Geometry check sheet. Reference: the model listing, model coordinates, mm. Face numbers are marked on the shaded views. A direction names the side the tool comes from. Round coordinates to 2 decimals unless told otherwise and drop trailing zeros. Loops run counter-clockwise (first coordinate to the right, second up) from the corner with the lowest first, then second, coordinate; pieces in that order, holes last. Notation, with made-up numbers: (-12, 68.5) - (-7, 68.5) arc R29 ccw to (-7, 100.5) - close; hole circle Ø7 at (75.5, -24.75). An arc over 180 degrees is marked (long way). Write item = value, one per line.
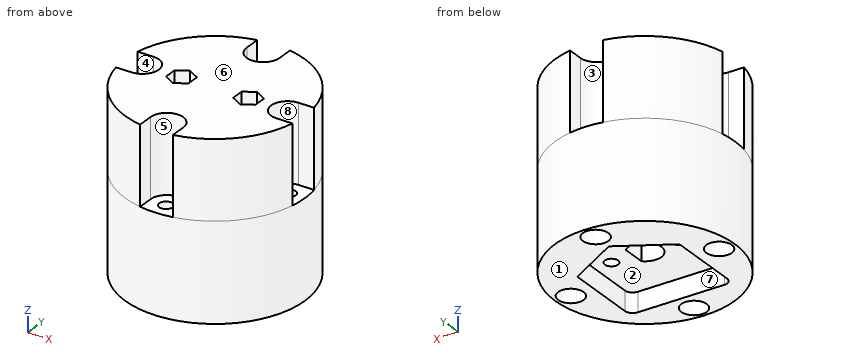
```python
from build123d import *

# Parameters (mm, degrees)
BOSS_EXTRUDE1_OUTLINE_R    = 16
BOSS_EXTRUDE1_DEPTH        = 15
SKETCH2_W                  = 7.4
SKETCH2_H                  = 24.742483552
CUT_EXTRUDE1_DEPTH         = 16.8
SKETCH3_R                  = 1.71
CUT_EXTRUDE2_DEPTH         = 70
BOSS_EXTRUDE2_DEPTH        = 20
BOSS_EXTRUDE2_DEPTH_BACK   = 5
SKETCH10_R                 = 23
SKETCH10_R_2               = 1.7
CUT_EXTRUDE4_DEPTH         = 25
SKETCH3_11_R               = 1.71
CUT_EXTRUDE5_DEPTH         = 55
CUT_EXTRUDE6_DEPTH         = 2.3
CUT_EXTRUDE6_DEPTH_BACK    = 0.7
SKETCH14_R                 = 12.3
BOSS_EXTRUDE3_START        = 20
BOSS_EXTRUDE3_DEPTH        = 20
SKETCH19_R                 = 16.2
CUT_EXTRUDE7_DEPTH         = 2.2
CUT_EXTRUDE8_START         = 35
CUT_EXTRUDE8_OUTLINE_R     = 1.7
CUT_EXTRUDE8_DEPTH         = 20
CUT_EXTRUDE9_START         = 2
CUT_EXTRUDE9_OUTLINE_R     = 16
CUT_EXTRUDE9_OUTLINE_R_2   = 15.484452344
CUT_EXTRUDE9_DEPTH         = 8
CUT_EXTRUDE9_START_2       = 10
CUT_EXTRUDE9_2_OUTLINE_R   = 3.25
CUT_EXTRUDE9_2_OUTLINE_R_2 = 1.7
CUT_EXTRUDE9_2_DEPTH       = 3
CUT_EXTRUDE10_DEPTH        = 3.6
SKETCH36_R                 = 15.484452344
CUT_EXTRUDE11_DEPTH        = 8
CUT_EXTRUDE13_DEPTH        = 5
CUT_EXTRUDE14_DEPTH        = 10
SKETCH39_R                 = 3.25
CUT_EXTRUDE15_DEPTH        = 5


# Read off the part's stored shape, not the designer's step: Boss-Extrude1, Cut-Extrude8, Cut-Extrude9
with BuildPart() as part:
    # Boss-Extrude1 outline → Boss-Extrude1 (new body)
    with BuildSketch(Plane(origin=(0, 0, 0), x_dir=(0, 1, 0), z_dir=(0, 0, 1))):
        Circle(BOSS_EXTRUDE1_OUTLINE_R)
    extrude(amount=BOSS_EXTRUDE1_DEPTH)

    # Sketch2 → Cut-Extrude1 (cut)
    with BuildSketch(Plane.ZY.offset(16)):
        with Locations((10.1, 0)):
            Rectangle(SKETCH2_W, SKETCH2_H)
    extrude(amount=-CUT_EXTRUDE1_DEPTH, mode=Mode.SUBTRACT)

    # Sketch3 → Cut-Extrude2 (cut)
    with BuildSketch(Plane(origin=(0, 0, 0), x_dir=(0, 1, 0), z_dir=(0, 0, 1))):
        with Locations((0, 8.6)):
            Circle(SKETCH3_R)
    extrude(amount=CUT_EXTRUDE2_DEPTH, mode=Mode.SUBTRACT)

    # Sketch10 → Boss-Extrude2 (add, two sides: drawn at the far end of the back side and taken through both)
    with BuildSketch(Plane(origin=(0, 0, 15), x_dir=(0, 1, 0), z_dir=(0, 0, 1)).offset(-BOSS_EXTRUDE2_DEPTH_BACK)):
        with Locations(Location((0, 0, 0), (0, 0, 270))):
            Circle(SKETCH10_R)
        with Locations(Location((0, 8.6, 0), (0, 0, 270))):
            Circle(SKETCH10_R_2, mode=Mode.SUBTRACT)
        with Locations(Location((0, 19, 0), (0, 0, 270))):
            Circle(SKETCH10_R_2, mode=Mode.SUBTRACT)
        with Locations(Location((18.999966339, -0.035764812, 0), (0, 0, 90))):
            Circle(SKETCH10_R_2, mode=Mode.SUBTRACT)
        with Locations(Location((0, -19, 0), (0, 0, 90))):
            Circle(SKETCH10_R_2, mode=Mode.SUBTRACT)
        with Locations(Location((-18.999966339, -0.035764812, 0), (0, 0, 270))):
            Circle(SKETCH10_R_2, mode=Mode.SUBTRACT)
        with Locations(Location((0, -8.6, 0), (0, 0, 270))):
            Circle(SKETCH10_R_2, mode=Mode.SUBTRACT)
    extrude(amount=BOSS_EXTRUDE2_DEPTH + BOSS_EXTRUDE2_DEPTH_BACK)

    # Sketch3<6> → Cut-Extrude4 (cut)
    with BuildSketch(Plane(origin=(0, 0, 0), x_dir=(0, 1, 0), z_dir=(0, 0, 1))):
        with BuildLine():
            Line((3, -2.939387691), (-3, -2.939387691))
            ThreePointArc((-3, -2.939387691), (0, 4.2), (3, -2.939387691))
        make_face()
    extrude(amount=CUT_EXTRUDE4_DEPTH, mode=Mode.SUBTRACT)

    # Sketch3<11> → Cut-Extrude5 (cut)
    with BuildSketch(Plane(origin=(0, 0, 0), x_dir=(0, 1, 0), z_dir=(0, 0, 1))):
        with Locations(Location((0, -8.6, 0), (0, 0, 90))):
            Circle(SKETCH3_11_R)
    extrude(amount=CUT_EXTRUDE5_DEPTH, mode=Mode.SUBTRACT)

    # Sketch14 → Cut-Extrude6 (cut, two sides: drawn at the far end of the back side and taken through both)
    with BuildSketch(Plane(origin=(0, 0, 7.5), x_dir=(0, 1, 0), z_dir=(0, 0, 1)).offset(-CUT_EXTRUDE6_DEPTH_BACK)):
        Circle(SKETCH14_R)
    extrude(amount=CUT_EXTRUDE6_DEPTH + CUT_EXTRUDE6_DEPTH_BACK, mode=Mode.SUBTRACT)

    # Sketch15 → Boss-Extrude3 (add)
    with BuildSketch(Plane(origin=(0, 0, 35), x_dir=(0, 1, 0), z_dir=(0, 0, 1)).offset(BOSS_EXTRUDE3_START)):
        with BuildLine():
            Line((-4.2, 18.6), (-4.2, 22.61327044))
            ThreePointArc((-4.2, 22.61327044), (-16.263455967, 16.263455967), (-22.61327044, 4.2))
            Line((-22.61327044, 4.2), (-18.6, 4.2))
            ThreePointArc((-18.6, 4.2), (-14.4, 0), (-18.6, -4.2))
            Line((-18.6, -4.2), (-22.61327044, -4.2))
            ThreePointArc((-22.61327044, -4.2), (-16.263455967, -16.263455967), (-4.2, -22.61327044))
            Line((-4.2, -22.61327044), (-4.2, -18.6))
            ThreePointArc((-4.2, -18.6), (0, -14.4), (4.2, -18.6))
            Line((4.2, -18.6), (4.2, -22.61327044))
            ThreePointArc((4.2, -22.61327044), (16.263455967, -16.263455967), (22.61327044, -4.2))
            Line((22.61327044, -4.2), (18.6, -4.2))
            ThreePointArc((18.6, -4.2), (14.4, 0), (18.6, 4.2))
            Line((18.6, 4.2), (22.61327044, 4.2))
            ThreePointArc((22.61327044, 4.2), (16.263455967, 16.263455967), (4.2, 22.61327044))
            Line((4.2, 22.61327044), (4.2, 18.6))
            ThreePointArc((4.2, 18.6), (0, 14.4), (-4.2, 18.6))
        make_face()
    extrude(amount=-BOSS_EXTRUDE3_DEPTH)

    # Sketch19 → Cut-Extrude7 (cut)
    with BuildSketch(Plane.YX.offset(0.2)):
        Circle(SKETCH19_R)
    extrude(amount=-CUT_EXTRUDE7_DEPTH, mode=Mode.SUBTRACT)

    # Cut-Extrude8 outline → Cut-Extrude8 (cut)
    with BuildSketch(Plane.XY.offset(CUT_EXTRUDE8_START)):
        with Locations((-8.6, 0)):
            Circle(CUT_EXTRUDE8_OUTLINE_R)
        with Locations((8.6, 0)):
            Circle(CUT_EXTRUDE8_OUTLINE_R)
    extrude(amount=CUT_EXTRUDE8_DEPTH, mode=Mode.SUBTRACT)

    # Sketch24 → CBORE for M3 SHCS1 (revolve, cut)
    with BuildSketch(Plane(origin=(0.035764812, 18.999966339, 10), x_dir=(0, 1, 0), z_dir=(1, 0, 0))):
        Polygon((0, 0), (0, 45), (1.7, 45), (1.7, 3), (3.25, 3), (3.25, 0), align=None)
    revolve(axis=Axis((0.035764812, 18.999966339, 3.65), (0, 0, 1)), mode=Mode.SUBTRACT)

    # Cut-Extrude9 outline → Cut-Extrude9 (cut)
    with BuildSketch(Plane.XY.offset(CUT_EXTRUDE9_START)):
        Circle(CUT_EXTRUDE9_OUTLINE_R)
        Circle(CUT_EXTRUDE9_OUTLINE_R_2, mode=Mode.SUBTRACT)
    extrude(amount=CUT_EXTRUDE9_DEPTH, mode=Mode.SUBTRACT)

    # Cut-Extrude9 2 outline → Cut-Extrude9 2 (cut)
    # profile 1 of 3: a face of its own
    with BuildSketch(Plane.XY.offset(CUT_EXTRUDE9_START_2)):
        with Locations((-19, 0)):
            Circle(CUT_EXTRUDE9_2_OUTLINE_R)
        with Locations((-19, 0)):
            Circle(CUT_EXTRUDE9_2_OUTLINE_R_2, mode=Mode.SUBTRACT)
    # profile 2 of 3: a face of its own
    with BuildSketch(Plane.XY.offset(CUT_EXTRUDE9_START_2)):
        with Locations((19, 0)):
            Circle(CUT_EXTRUDE9_2_OUTLINE_R)
        with Locations((19, 0)):
            Circle(CUT_EXTRUDE9_2_OUTLINE_R_2, mode=Mode.SUBTRACT)
    # profile 3 of 3: a face of its own
    with BuildSketch(Plane.XY.offset(CUT_EXTRUDE9_START_2)):
        with Locations((0.035764812, -18.999966339)):
            Circle(CUT_EXTRUDE9_2_OUTLINE_R)
        with Locations((0.035764812, -18.999966339)):
            Circle(CUT_EXTRUDE9_2_OUTLINE_R_2, mode=Mode.SUBTRACT)
    extrude(amount=CUT_EXTRUDE9_2_DEPTH, mode=Mode.SUBTRACT)

    # Sketch31 → Cut-Extrude10 (cut)
    with BuildSketch(Plane(origin=(0, 0, 10), x_dir=(0, 1, 0), z_dir=(0, 0, 1))):
        with BuildLine():
            Line((-12.4, 0), (12.4, 0))
            ThreePointArc((12.4, 0), (0, -12.4), (-12.4, 0))
        make_face()
    extrude(amount=-CUT_EXTRUDE10_DEPTH, mode=Mode.SUBTRACT)

    # Sketch36 → Cut-Extrude11 (cut)
    with BuildSketch(Plane(origin=(0, 0, 2), x_dir=(0, 1, 0), z_dir=(0, 0, 1))):
        Circle(SKETCH36_R)
    extrude(amount=CUT_EXTRUDE11_DEPTH, mode=Mode.SUBTRACT)

    # Sketch37 → Cut-Extrude13 (cut)
    with BuildSketch(Plane(origin=(0, 0, 15), x_dir=(0, 1, 0), z_dir=(0, 0, 1))):
        with BuildLine():
            Line((6.408587988, -13.1), (13.971876514, 0))
            Line((13.971876514, 0), (6.408587988, 13.1))
            Line((6.408587988, 13.1), (-11.971876514, 13.1))
            ThreePointArc((-11.971876514, 13.1), (-13.386090077, 12.514213562), (-13.971876514, 11.1))
            Line((-13.971876514, 11.1), (-13.971876514, -11.1))
            ThreePointArc((-13.971876514, -11.1), (-13.386090077, -12.514213562), (-11.971876514, -13.1))
            Line((-11.971876514, -13.1), (6.408587988, -13.1))
        make_face()
    extrude(amount=-CUT_EXTRUDE13_DEPTH, mode=Mode.SUBTRACT)

    # Sketch38 → Cut-Extrude14 (cut)
    with BuildSketch(Plane(origin=(0, 0, 55), x_dir=(0, 1, 0), z_dir=(0, 0, 1))):
        Polygon((3.290896534, 8.6), (1.645448267, 11.45), (-1.645448267, 11.45), (-3.290896534, 8.6), (-1.645448267, 5.75), (1.645448267, 5.75), align=None)
        Polygon((3.290896534, -8.6), (1.645448267, -5.75), (-1.645448267, -5.75), (-3.290896534, -8.6), (-1.645448267, -11.45), (1.645448267, -11.45), align=None)
    extrude(amount=-CUT_EXTRUDE14_DEPTH, mode=Mode.SUBTRACT)

    # Sketch39 → Cut-Extrude15 (cut)
    with BuildSketch(Plane(origin=(0, 0, 10), x_dir=(0, 1, 0), z_dir=(0, 0, 1))):
        with Locations(Location((0, 19, 0), (0, 0, 90))):
            Circle(SKETCH39_R)
        with Locations(Location((-18.999966339, -0.035764812, 0), (0, 0, 90))):
            Circle(SKETCH39_R)
        with Locations(Location((0, -19, 0), (0, 0, 90))):
            Circle(SKETCH39_R)
        with Locations(Location((18.999966339, -0.035764812, 0), (0, 0, 90))):
            Circle(SKETCH39_R)
    extrude(amount=CUT_EXTRUDE15_DEPTH, mode=Mode.SUBTRACT)


solid = part.part
```
(1) Set-up check for the marked faces 4, 5, 6, 7 and 8: record each of +Z, -Z, +X, -X, +Y, -Y from which the full face is reachable in a straight line by a thin tool's end or side.
Answers follow:
face_4 = +Z, -X
face_5 = +Z, -Y
face_6 = +Z, +X, -X, +Y, -Y
face_7 = -Z
face_8 = +Z, +X
(2) Scan lines: L1, parallel to Y at x = 0, z = 22; L2, parallel to Y at x = 0, z = 52; L3, parallel to Z at x = -8.5, y = 5. Record each from-to range of solid material in increasing order. Write a range as [from, to].
Answers follow:
L1 = [-23, -20.7], [-17.3, -4.2], [4.2, 17.3], [20.7, 23]
L2 = [-14.4, 14.4]
L3 = [15, 55]
(3) Mould release check, pull along Y, two halves, no side actions. Record for the marked faces 1, 2 and 3: pulls with the +Y half, pulls with the -Y half, needs draft (parallel to the pull), parting line crosses it, or undercut.
Answers follow:
face_1 = needs draft
face_2 = undercut
face_3 = pulls with the +Y half
(4) Section check D-D (z = 36). Enter the section's corners in (x, y), then the cut area to 3 significant figures.
Answers follow:
outline = (-22.61, -4.2) arc R23 ccw to (-4.2, -22.61) - (-4.2, -18.6) arc R4.2 cw to (4.2, -18.6) - (4.2, -22.61) arc R23 ccw to (22.61, -4.2) - (18.6, -4.2) arc R4.2 cw to (18.6, 4.2) - (22.61, 4.2) arc R23 ccw to (4.2, 22.61) - (4.2, 18.6) arc R4.2 cw to (-4.2, 18.6) - (-4.2, 22.61) arc R23 ccw to (-22.61, 4.2) - (-18.6, 4.2) arc R4.2 cw to (-18.6, -4.2) - close; hole circle Ø3.4 at (-8.6, 0); hole circle Ø3.4 at (8.6, 0)
area = 1,390 mm²
(5) Section check C-C (z = 28). Enter the section's corners in (x, y).
Answers follow:
outline = circle Ø46 at (0, 0); hole circle Ø3.4 at (-19, 0); hole circle Ø3.4 at (-8.6, 0); hole circle Ø3.4 at (0.04, -19); hole circle Ø3.4 at (0.04, 19); hole circle Ø3.42 at (8.6, 0); hole circle Ø3.4 at (19, 0)
(6) Section check A-A (z = 49). Enter the section's corners in (x, y), then the cut area to 3 significant figures.
Answers follow:
outline = (-22.61, -4.2) arc R23 ccw to (-4.2, -22.61) - (-4.2, -18.6) arc R4.2 cw to (4.2, -18.6) - (4.2, -22.61) arc R23 ccw to (22.61, -4.2) - (18.6, -4.2) arc R4.2 cw to (18.6, 4.2) - (22.61, 4.2) arc R23 ccw to (4.2, 22.61) - (4.2, 18.6) arc R4.2 cw to (-4.2, 18.6) - (-4.2, 22.61) arc R23 ccw to (-22.61, 4.2) - (-18.6, 4.2) arc R4.2 cw to (-18.6, -4.2) - close; hole (-11.45, -1.65) - (-8.6, -3.29) - (-5.75, -1.65) - (-5.75, 1.65) - (-8.6, 3.29) - (-11.45, 1.65) - close; hole (5.75, -1.65) - (8.6, -3.29) - (11.45, -1.65) - (11.45, 1.65) - (8.6, 3.29) - (5.75, 1.65) - close
area = 1,350 mm²
(7) Section check B-B (y = 0). State how many separate pieces and enclosed holes the cut face has, then the cut area to 3 significant figures.
Answers follow:
separate_pieces = 5
enclosed_holes = 0
area = 1,000 mm²
(8) Gauge pin test, flat ends, axial feed: pin 1 (4 mm diameter, centred on y = -5.5, z = 42, fed in from -X); pin 2 (3 mm diameter, centred on y = -21, z = 48.5, fed in from -X); pin 3 (1 mm diameter, centred on y = -15, z = 28.5, fed in from -X); pin 4 (3 mm diameter, centred on x = 19, y = 0, fed in from -Z). Record the tip position at first contact, or that the pin passes through.
Answers follow:
pin_1 = -22.61
pin_2 = -12.2
pin_3 = -17.85
pin_4 = through
